The listing builds one solid part. Answer for the finished solid, in the listing's coordinates (mm). A direction names the side the tool comes from. Give positions to 0.01 mm unless a question says otherwise; leave off trailing zeros. Write each loop counter-clockwise with the first axis right and the second up, starting at its lowest first coordinate (ties: lowest second). Pieces come first, ordered by that corner, then holes. Notation, with made-up numbers: M -10,83.25 L 44,83.25 A12 cw 44,87.25 Z; hole C 82.25,13 d1. An arc over 180 degrees is marked long. Return JSON: item names as keys, results as strings.
Autodesk Inventor part; units mm, degrees
ref_plane "YZ Plane" through (0, 0, 0) normal (1, 0, 0) x (0, 1, 0)
ref_plane "XZ Plane" through (0, 0, 0) normal (0, 1, 0) x (-1, 0, 0)
ref_plane "XY Plane" through (0, 0, 0) normal (0, 0, 1) x (1, 0, 0)
sketch "Sketch1" plane through (0, 0, 0) normal (0, 0, 1) x (1, 0, 0)
  line L0 (-31.9903, -7.2804) -> (-1.9903, -7.2804)
  line L1 (-1.9903, -7.2804) -> (-1.9903, 22.7196)
  line L2 (-1.9903, 22.7196) -> (-31.9903, 22.7196)
  line L3 (-31.9903, -7.2804) -> (-31.9903, 22.7196)
  line L4 (-30.2903, 22.7196) -> (-30.2903, -7.2804)
  line L5 (-31.9903, -5.5804) -> (-1.9903, -5.5804)
  line L6 (-3.6903, 22.7196) -> (-3.6903, -7.2804)
  line L7 (-31.9903, 21.0196) -> (-1.9903, 21.0196)
  point P0 (0, 0)
  point P1 (0, 0)
  point P2 (-3.6903, 21.0196)
  point P3 (-30.2903, 21.0196)
  point P4 (-30.2903, -5.5804)
  point P5 (-3.6903, -5.5804)
  dimension "d0" = 30
  dimension "d1" = 30
  dimension "d2" = 1.7
  dimension "d3" = 1.7
  dimension "d4" = 1.7
  dimension "d5" = 1.7
extrude "Extrusion1" add sketch "Sketch1" against normal blind 119.543
extrude "Extrusion2" cut sketch "Sketch1" against normal blind 119.543 contours L4 L7 L6 L5
properties part number "Cablecanal Ranurado 30x30 L=115  mm" material "PVC-Piping"
Item 1: Determine the mould class of faces 3 (the flat face through (-1.99, 8, -59)), 4 (the flat face through (-17, -7.28, -59)), 5 (the flat face through (-3.69, 8, -59)) for opening direction Y: +Y half, -Y half, draft (parallel to the pull), parting line (faces both ways), or undercut.
Geometry results:
{"face 3": "draft", "face 4": "-Y half", "face 5": "undercut"}
Item 2: A cutting plane is placed at A-A, the plane x = -12. Write down the section's boundary in (y, z), plus the area to 3 significant figures.
Geometry results:
{"outline": "M -7.28,-119.54 L -5.58,-119.54 L -5.58,0 L -7.28,0 Z; M 21.02,-119.54 L 22.72,-119.54 L 22.72,0 L 21.02,0 Z", "area": "406 mm2"}
Item 3: A cutting plane is placed at C-C, the plane z = -78.5. Write down the section's boundary in (x, y).
Geometry results:
{"outline": "M -31.99,-7.28 L -1.99,-7.28 L -1.99,22.72 L -31.99,22.72 Z; hole M -30.29,-5.58 L -3.69,-5.58 L -3.69,21.02 L -30.29,21.02 Z"}
Item 4: A cutting plane is placed at B-B, the plane y = 14.5. Write down the section's boundary in (x, z), plus the area to 3 significant figures.
Geometry results:
{"outline": "M -31.99,-119.54 L -30.29,-119.54 L -30.29,0 L -31.99,0 Z; M -3.69,-119.54 L -1.99,-119.54 L -1.99,0 L -3.69,0 Z", "area": "406 mm2"}
Item 5: Which of the six approach directions +Z, -Z, +X, -X, +Y, -Y give full straight-line access (tool end or side, diameter ignored) to faces 1 (the flat face through (-17, -5.58, -59)), 2 (the flat face through (-17, 22.72, -59))?
Geometry results:
{"face 1": "+Z, -Z", "face 2": "+Z, -Z, +X, -X, +Y"}
Item 6: Find the intervals of material crossed by line 1 (X direction, y = 12.5, z = -65); line 2 (Y direction, x = -15.5, z = -30), in increasing order.
Geometry results:
{"line 1": "x = -31.99 to -30.29, -3.69 to -1.99", "line 2": "y = -7.28 to -5.58, 21.02 to 22.72"}
